Source: CAD feature listing. Evaluate the final solid. Frame: model axes, mm. Round coordinates to 2 decimals unless told otherwise and drop trailing zeros. Return JSON: item names as keys, results as strings. Group by question number.
from build123d import *

# Parameters (mm, degrees)
CROQUIS4_R                 = 2.5
MIEMBRO_ESTRUCTURAL1_DEPTH = 440


with BuildPart() as part:
    # Croquis4 → Miembro estructural1 (new body)
    with BuildSketch(Plane.XY.offset(-220)):
        with BuildLine():
            Line((-19, -10), (-15.410285706, -10))
            Line((-15.410285706, -10), (-13.270710678, -7.860424973))
            ThreePointArc((-13.270710678, -7.860424973), (-13.249033403, -7.751445951), (-13.341421356, -7.689714294))
            Line((-13.341421356, -7.689714294), (-16.358578644, -7.689714294))
            ThreePointArc((-16.358578644, -7.689714294), (-16.450966597, -7.627982638), (-16.429289322, -7.519003616))
            Line((-16.429289322, -7.519003616), (-13.629289322, -4.719003616))
            ThreePointArc((-13.629289322, -4.719003616), (-13.596846987, -4.697326341), (-13.558578644, -4.689714294))
            Line((-13.558578644, -4.689714294), (-6.441421356, -4.689714294))
            ThreePointArc((-6.441421356, -4.689714294), (-6.403153013, -4.697326341), (-6.370710678, -4.719003616))
            Line((-6.370710678, -4.719003616), (-3.570710678, -7.519003616))
            ThreePointArc((-3.570710678, -7.519003616), (-3.549033403, -7.627982638), (-3.641421356, -7.689714294))
            Line((-3.641421356, -7.689714294), (-6.658578644, -7.689714294))
            ThreePointArc((-6.658578644, -7.689714294), (-6.750966597, -7.751445951), (-6.729289322, -7.860424973))
            Line((-6.729289322, -7.860424973), (-4.589714294, -10))
            Line((-4.589714294, -10), (4.589714294, -10))
            Line((4.589714294, -10), (6.729289322, -7.860424973))
            ThreePointArc((6.729289322, -7.860424973), (6.750966597, -7.751445951), (6.658578644, -7.689714294))
            Line((6.658578644, -7.689714294), (3.641421356, -7.689714294))
            ThreePointArc((3.641421356, -7.689714294), (3.549033403, -7.627982638), (3.570710678, -7.519003616))
            Line((3.570710678, -7.519003616), (6.370710678, -4.719003616))
            ThreePointArc((6.370710678, -4.719003616), (6.403153013, -4.697326341), (6.441421356, -4.689714294))
            Line((6.441421356, -4.689714294), (13.558578644, -4.689714294))
            ThreePointArc((13.558578644, -4.689714294), (13.596846987, -4.697326341), (13.629289322, -4.719003616))
            Line((13.629289322, -4.719003616), (16.429289322, -7.519003616))
            ThreePointArc((16.429289322, -7.519003616), (16.450966597, -7.627982638), (16.358578644, -7.689714294))
            Line((16.358578644, -7.689714294), (13.341421356, -7.689714294))
            ThreePointArc((13.341421356, -7.689714294), (13.249033403, -7.751445951), (13.270710678, -7.860424973))
            Line((13.270710678, -7.860424973), (15.410285706, -10))
            Line((15.410285706, -10), (19, -10))
            ThreePointArc((19, -10), (19.707106781, -9.707106781), (20, -9))
            Line((20, -9), (20, -5.410285706))
            Line((20, -5.410285706), (17.860424973, -3.270710678))
            ThreePointArc((17.860424973, -3.270710678), (17.751445951, -3.249033403), (17.689714294, -3.341421356))
            Line((17.689714294, -3.341421356), (17.689714294, -6.358578644))
            ThreePointArc((17.689714294, -6.358578644), (17.627982638, -6.450966597), (17.519003616, -6.429289322))
            Line((17.519003616, -6.429289322), (14.719003616, -3.629289322))
            ThreePointArc((14.719003616, -3.629289322), (14.697326341, -3.596846987), (14.689714294, -3.558578644))
            Line((14.689714294, -3.558578644), (14.689714294, 3.558578644))
            ThreePointArc((14.689714294, 3.558578644), (14.697326341, 3.596846987), (14.719003616, 3.629289322))
            Line((14.719003616, 3.629289322), (17.519003616, 6.429289322))
            ThreePointArc((17.519003616, 6.429289322), (17.627982638, 6.450966597), (17.689714294, 6.358578644))
            Line((17.689714294, 6.358578644), (17.689714294, 3.341421356))
            ThreePointArc((17.689714294, 3.341421356), (17.751445951, 3.249033403), (17.860424973, 3.270710678))
            Line((17.860424973, 3.270710678), (20, 5.410285706))
            Line((20, 5.410285706), (20, 9))
            ThreePointArc((20, 9), (19.707106781, 9.707106781), (19, 10))
            Line((19, 10), (15.410285706, 10))
            Line((15.410285706, 10), (13.270710678, 7.860424973))
            ThreePointArc((13.270710678, 7.860424973), (13.249033403, 7.751445951), (13.341421356, 7.689714294))
            Line((13.341421356, 7.689714294), (16.358578644, 7.689714294))
            ThreePointArc((16.358578644, 7.689714294), (16.450966597, 7.627982638), (16.429289322, 7.519003616))
            Line((16.429289322, 7.519003616), (13.629289322, 4.719003616))
            ThreePointArc((13.629289322, 4.719003616), (13.596846987, 4.697326341), (13.558578644, 4.689714294))
            Line((13.558578644, 4.689714294), (6.441421356, 4.689714294))
            ThreePointArc((6.441421356, 4.689714294), (6.403153013, 4.697326341), (6.370710678, 4.719003616))
            Line((6.370710678, 4.719003616), (3.570710678, 7.519003616))
            ThreePointArc((3.570710678, 7.519003616), (3.549033403, 7.627982638), (3.641421356, 7.689714294))
            Line((3.641421356, 7.689714294), (6.658578644, 7.689714294))
            ThreePointArc((6.658578644, 7.689714294), (6.750966597, 7.751445951), (6.729289322, 7.860424973))
            Line((6.729289322, 7.860424973), (4.589714294, 10))
            Line((4.589714294, 10), (-4.589714294, 10))
            Line((-4.589714294, 10), (-6.729289322, 7.860424973))
            ThreePointArc((-6.729289322, 7.860424973), (-6.750966597, 7.751445951), (-6.658578644, 7.689714294))
            Line((-6.658578644, 7.689714294), (-3.641421356, 7.689714294))
            ThreePointArc((-3.641421356, 7.689714294), (-3.549033403, 7.627982638), (-3.570710678, 7.519003616))
            Line((-3.570710678, 7.519003616), (-6.370710678, 4.719003616))
            ThreePointArc((-6.370710678, 4.719003616), (-6.403153013, 4.697326341), (-6.441421356, 4.689714294))
            Line((-6.441421356, 4.689714294), (-13.558578644, 4.689714294))
            ThreePointArc((-13.558578644, 4.689714294), (-13.596846987, 4.697326341), (-13.629289322, 4.719003616))
            Line((-13.629289322, 4.719003616), (-16.429289322, 7.519003616))
            ThreePointArc((-16.429289322, 7.519003616), (-16.450966597, 7.627982638), (-16.358578644, 7.689714294))
            Line((-16.358578644, 7.689714294), (-13.341421356, 7.689714294))
            ThreePointArc((-13.341421356, 7.689714294), (-13.249033403, 7.751445951), (-13.270710678, 7.860424973))
            Line((-13.270710678, 7.860424973), (-15.410285706, 10))
            Line((-15.410285706, 10), (-19, 10))
            ThreePointArc((-19, 10), (-19.707106781, 9.707106781), (-20, 9))
            Line((-20, 9), (-20, 5.410285706))
            Line((-20, 5.410285706), (-17.860424973, 3.270710678))
            ThreePointArc((-17.860424973, 3.270710678), (-17.751445951, 3.249033403), (-17.689714294, 3.341421356))
            Line((-17.689714294, 3.341421356), (-17.689714294, 6.358578644))
            ThreePointArc((-17.689714294, 6.358578644), (-17.627982638, 6.450966597), (-17.519003616, 6.429289322))
            Line((-17.519003616, 6.429289322), (-14.719003616, 3.629289322))
            ThreePointArc((-14.719003616, 3.629289322), (-14.697326341, 3.596846987), (-14.689714294, 3.558578644))
            Line((-14.689714294, 3.558578644), (-14.689714294, -3.558578644))
            ThreePointArc((-14.689714294, -3.558578644), (-14.697326341, -3.596846987), (-14.719003616, -3.629289322))
            Line((-14.719003616, -3.629289322), (-17.519003616, -6.429289322))
            ThreePointArc((-17.519003616, -6.429289322), (-17.627982638, -6.450966597), (-17.689714294, -6.358578644))
            Line((-17.689714294, -6.358578644), (-17.689714294, -3.341421356))
            ThreePointArc((-17.689714294, -3.341421356), (-17.751445951, -3.249033403), (-17.860424973, -3.270710678))
            Line((-17.860424973, -3.270710678), (-20, -5.410285706))
            Line((-20, -5.410285706), (-20, -9))
            ThreePointArc((-20, -9), (-19.707106781, -9.707106781), (-19, -10))
        make_face()
        with Locations((-10, 0)):
            Circle(CROQUIS4_R, mode=Mode.SUBTRACT)
        with Locations((10, 0)):
            Circle(CROQUIS4_R, mode=Mode.SUBTRACT)
        with BuildLine():
            Line((-2.480996384, 6.429289322), (-5.280996384, 3.629289322))
            ThreePointArc((-5.280996384, 3.629289322), (-5.302673659, 3.596846987), (-5.310285706, 3.558578644))
            Line((-5.310285706, 3.558578644), (-5.310285706, -3.558578644))
            ThreePointArc((-5.310285706, -3.558578644), (-5.302673659, -3.596846987), (-5.280996384, -3.629289322))
            Line((-5.280996384, -3.629289322), (-2.480996384, -6.429289322))
            Line((-2.480996384, -6.429289322), (-1.220571411, -7.689714294))
            Line((-1.220571411, -7.689714294), (1.220571411, -7.689714294))
            Line((1.220571411, -7.689714294), (2.480996384, -6.429289322))
            Line((2.480996384, -6.429289322), (5.280996384, -3.629289322))
            ThreePointArc((5.280996384, -3.629289322), (5.302673659, -3.596846987), (5.310285706, -3.558578644))
            Line((5.310285706, -3.558578644), (5.310285706, 3.558578644))
            ThreePointArc((5.310285706, 3.558578644), (5.302673659, 3.596846987), (5.280996384, 3.629289322))
            Line((5.280996384, 3.629289322), (2.480996384, 6.429289322))
            Line((2.480996384, 6.429289322), (1.220571411, 7.689714294))
            Line((1.220571411, 7.689714294), (-1.220571411, 7.689714294))
            Line((-1.220571411, 7.689714294), (-2.480996384, 6.429289322))
        make_face(mode=Mode.SUBTRACT)
    extrude(amount=MIEMBRO_ESTRUCTURAL1_DEPTH)


solid = part.part
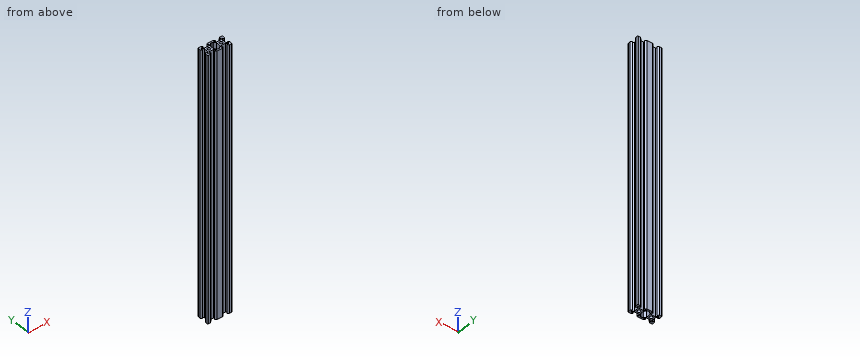
Item 1: Cut plane A-A on z = -174.5. Give the number of separate pieces and of enclosed holes in the cut face, and give its area (3 significant figures).
Item 2: Material intervals for probe 1 along X at (y, z) = (-6.5, -202); probe 2 along Y at (x, z) = (-3.5, -183.5); probe 3 along Y at (x, z) = (10, 85), sorted ascending.
Item 3: First-contact query: pin 1 Ø2 at (y, z) = (0, 71) entering from -X; pin 2 Ø2 at (x, z) = (11, -8) entering from +Y; pin 3 Ø2 at (y, z) = (-0.5, 4.5) entering from +X. Flat tips, straight axial feed; report the tip coordinate or a pass-through.
Here are the results:
{
 "1": {"separate pieces": "1", "enclosed holes": "3", "area": "328 mm^2"},
 "2": {"probe 1": "x = -20 to -15.41, -4.59 to -2.41, 2.41 to 4.59, 15.41 to 20", "probe 2": "y = -10 to -5.41, 5.41 to 10", "probe 3": "y = -4.69 to -2.5, 2.5 to 4.69"},
 "3": {"pin 1": "stops at x = -14.69", "pin 2": "stops at y = 4.69", "pin 3": "stops at x = 14.69"}
}
